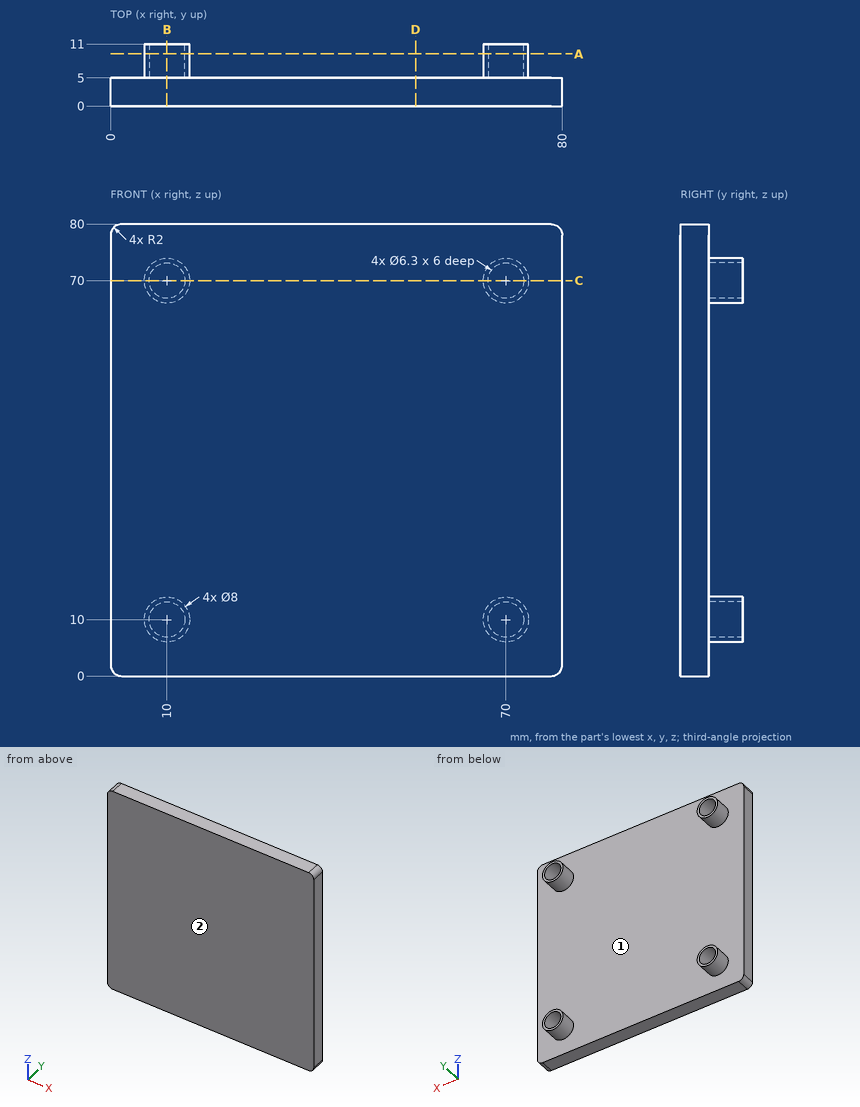
Job drawing, mm, ordinate dimensions from the low corner. One solid piece. A direction names the side the tool comes from. Round coordinates to 2 decimals unless told otherwise and drop trailing zeros. Write each loop counter-clockwise with the first axis right and the second up, starting at its lowest first coordinate (ties: lowest second). Pieces come first, ordered by that corner, then holes.
1) Drill centre lines: probe 1 along X at (y, z) = (9.05, 10); probe 2 along Z at (x, y) = (67.5, 10.75). Where is each one in solid material? Low to high.
2) Pin check, flat tips, straight feed: pin 1 (3 mm diameter, centred on x = 65.5, y = 7.5, fed in from +Z); pin 2 (3 mm diameter, centred on x = 71, z = 69.5, fed in from +Y). Stop position of each tip, or through.
3) Band-saw the part on A-A, the plane y = 9.25. List the corners of the cut face in (x, z), and give its area (3 significant figures).
4) Band-saw the part on C-C, the plane z = 70. List the corners of the cut face in (x, y).
5) Band-saw the part on B-B, the plane x = 10. List the corners of the cut face in (y, z), and give its area (3 significant figures).
6) 3-axis set-ups, long thin cutter, end or side, ignore diameter. For the marked faces 1 and 2: which of +Z, -Z, +X, -X, +Y, -Y reach the whole face in a straight line?
7) Band-saw the part on D-D, the plane x = 54. List the corners of the cut face in (y, z), and give its area (3 significant figures).
Ans:
1. probe 1: x = 6 to 6.85, 13.15 to 14, 66 to 66.85, 73.15 to 74
1. probe 2: z = 6.88 to 8.08, 11.92 to 13.12, 66.88 to 68.08, 71.92 to 73.12
2. pin 1: stops at z = 72.65
2. pin 2: stops at y = 5
3. outline: circle Ø8 at (10, 10); circle Ø8 at (10, 70); circle Ø8 at (70, 10); circle Ø8 at (70, 70); hole circle Ø6.3 at (10, 10); hole circle Ø6.3 at (10, 70); hole circle Ø6.3 at (70, 10); hole circle Ø6.3 at (70, 70)
3. area: 76.4 mm2
4. outline: (0, 0) - (80, 0) - (80, 5) - (74, 5) - (74, 11) - (73.15, 11) - (73.15, 5) - (66.85, 5) - (66.85, 11) - (66, 11) - (66, 5) - (14, 5) - (14, 11) - (13.15, 11) - (13.15, 5) - (6.85, 5) - (6.85, 11) - (6, 11) - (6, 5) - (0, 5) - close
5. outline: (0, 0) - (5, 0) - (5, 6) - (11, 6) - (11, 6.85) - (5, 6.85) - (5, 13.15) - (11, 13.15) - (11, 14) - (5, 14) - (5, 66) - (11, 66) - (11, 66.85) - (5, 66.85) - (5, 73.15) - (11, 73.15) - (11, 74) - (5, 74) - (5, 80) - (0, 80) - close
5. area: 420 mm2
6. face 1: +Y
6. face 2: +Z, -Z, +X, -X, -Y
7. outline: (0, 0) - (5, 0) - (5, 80) - (0, 80) - close
7. area: 400 mm2
